Verification items for this drawing (mm, ordinates from the low corner). A direction names the side the tool comes from. Coordinates: 2 decimals unless noted, no trailing zeros. Write each loop counter-clockwise with the first axis right and the second up, starting at its lowest first coordinate (ties: lowest second). Pieces come first, ordered by that corner, then holes. Notation, with made-up numbers: (-35.5, -6) -> (-18.5, -6) arc R17 ccw to (-18.5, 27) -> close; hole circle Ø8 at (72.25, 89.25). An arc over 180 degrees is marked (long way). One line per item, written item: value. Start each with the question number.
1) Sectioned sample at C-C on x = 75. Enter the section's corners in (y, z), plus the area to 3 significant figures.
2) Sectioned sample at D-D on z = 230. Enter the section's corners in (x, y).
3) Gauge pin test, flat ends, axial feed: P1, Ø12, axis at x = 352, z = 212, coming from the -Y side; P2, Ø6, axis at y = 133, z = 157, coming from the -X side; P3, Ø1.5, axis at y = 175.5, z = 205.5, coming from the +X side; P4, Ø20, axis at x = 575, z = 187.5, coming from the +Y side. Record the tip position at first contact, or that the pin passes through.
4) Sectioned sample at A-A on x = 325. Enter the section's corners in (y, z).
5) Sectioned sample at B-B on z = 187.5. Enter the section's corners in (x, y), plus the area to 3 significant figures.
6) Set-up check for the marked faces 1, 2 and 3: record each of +Z, -Z, +X, -X, +Y, -Y from which the full face is reachable in a straight line by a thin tool's end or side.
7) Scan lines: line 1 along Z through (x, y) = (75, 259); line 2 along Y through (x, z) = (589.5, 101.5); line 3 along X through (y, z) = (118, 221). Record each from-to range of solid material in increasing order. Write a range as [from, to].
8) Draft check along X on the marked faces 4, 5 and 6. Enter one of: +X half, -X half, draft (parallel to the pull), parting line (faces both ways), or undercut.
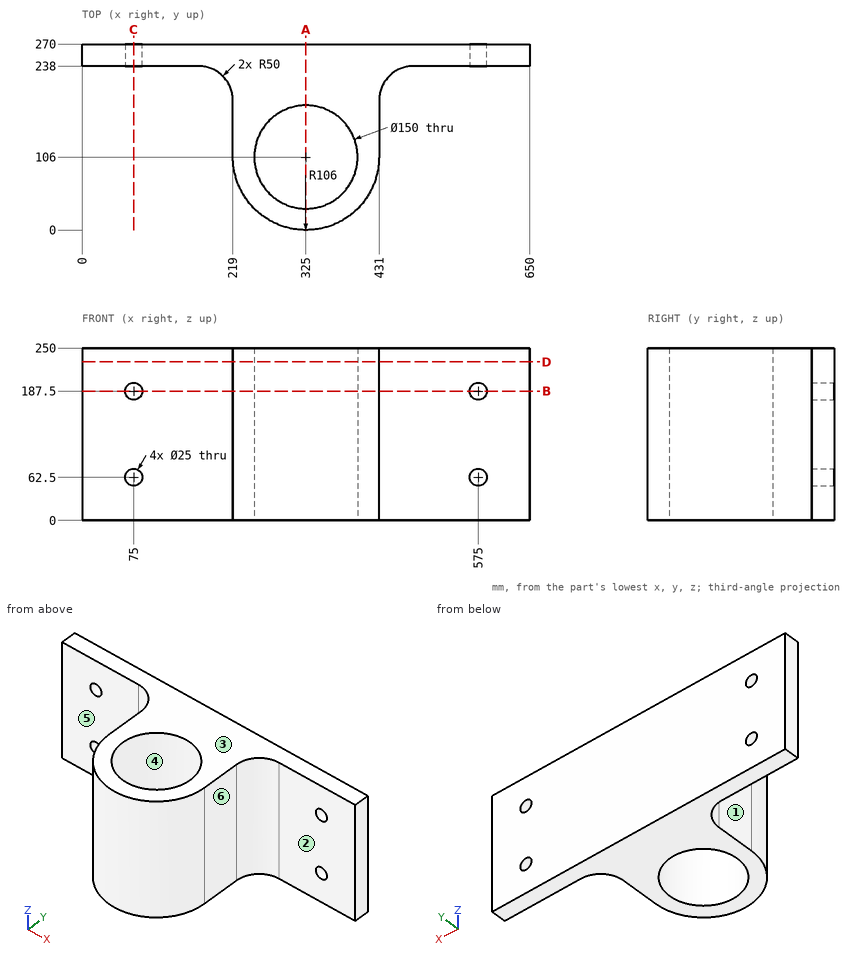
Answers:
1. outline: (238, 0) -> (270, 0) -> (270, 50) -> (238, 50) -> close; (238, 75) -> (270, 75) -> (270, 175) -> (238, 175) -> close; (238, 200) -> (270, 200) -> (270, 250) -> (238, 250) -> close
1. area: 6,400 mm2
2. outline: (0, 238) -> (169, 238) arc R50 cw to (219, 188) -> (219, 106) arc R106 ccw to (431, 106) -> (431, 188) arc R50 cw to (481, 238) -> (650, 238) -> (650, 270) -> (0, 270) -> close; hole circle Ø150 at (325, 106)
3. P1: stops at y = 2.1
3. P2: stops at x = 219
3. P3: stops at x = 431
3. P4: passes through
4. outline: (0, 0) -> (31, 0) -> (31, 250) -> (0, 250) -> close; (181, 0) -> (270, 0) -> (270, 250) -> (181, 250) -> close
5. outline: (0, 238) -> (62.5, 238) -> (62.5, 270) -> (0, 270) -> close; (87.5, 238) -> (169, 238) arc R50 cw to (219, 188) -> (219, 106) arc R106 ccw to (431, 106) -> (431, 188) arc R50 cw to (481, 238) -> (562.5, 238) -> (562.5, 270) -> (87.5, 270) -> close; (587.5, 238) -> (650, 238) -> (650, 270) -> (587.5, 270) -> close; hole circle Ø150 at (325, 106)
5. area: 48,200 mm2
6. face 1: +Z, -Z, -X, -Y
6. face 2: +Z, -Z, +X, -Y
6. face 3: +Z, +X, -X, +Y, -Y
7. line 1: z = [0, 50], [75, 175], [200, 250]
7. line 2: y = [238, 270]
7. line 3: x = [219, 250.97], [399.03, 431]
8. face 4: undercut
8. face 5: draft
8. face 6: +X half
